Build history of the part. All positions in model axes, mm. A direction names the side the tool comes from. Give positions to 0.01 mm unless a question says otherwise; leave off trailing zeros. Order: outer loops, then holes, each group sorted by start corner. A loop starts at its lowest first (then second) coordinate and runs counter-clockwise, first axis right, second up. Notation, with made-up numbers: (68, 29.25) - (123, 29.25) arc R33 ccw to (123, 61.25) - close; hole circle Ø11 at (48.25, 28). An arc over 180 degrees is marked (long way). Write each question's results on one line, items separated by ' | '. Start each with the question number.
1) Cut at B-B on y = 35. List the corners of the cut face in (x, z).
2) Two-plate mould, pull along Y, no slides. Class faces 1 (the face through (54, 0, -16)), 2 (the face through (53, 39.37, 2)), 3 (the face through (50.78, 23.7, 1.88)): +Y half, -Y half, draft (parallel to the pull), parting line (faces both ways), or undercut.
3) Drill centre lines: line 1 along Y through (x, z) = (53.34, 2.1); line 2 along Z through (x, y) = (18, 6). Where is each one in solid material? Low to high. Write a range as from..to.
4) Drop flat-ended pins along their axis: pin 1 Ø8 at (x, y) = (25.5, 24) entering from -Z; pin 2 Ø1 at (x, z) = (41, -31) entering from +Y. Give the stop position or say it passes through.
5) Cut at C-C on x = 7.5. List the corners of the cut face in (y, z).
6) Cut at A-A on x = 53.34. List the corners of the cut face in (y, z).
7) Tool access for faces 4 (the face through (0, 10.8, 0.3)), 5 (the face through (53, 25, 0)): list every direction of +Z, -Z, +X, -X, +Y, -Y with a clear straight run to the whole face (end or side of a thin tool).
Autodesk Inventor part; units mm, degrees
ref_plane "YZ Plane" through (0, 0, 0) normal (1, 0, 0) x (0, 1, 0)
ref_plane "XZ Plane" through (0, 0, 0) normal (0, 1, 0) x (-1, 0, 0)
ref_plane "XY Plane" through (0, 0, 0) normal (0, 0, 1) x (1, 0, 0)
sketch "Sketch1" plane through (0, 0, 0) normal (0, 1, 0) x (-1, 0, 0)
  line L0 (0, 0) -> (0, -35.56)
  line L1 (0, -35.56) -> (-106.68, -35.56)
  line L2 (-106.68, -35.56) -> (-106.68, 0)
  line L3 (0, 0) -> (0, 3.81)
  line L4 (0, 3.81) -> (-106.68, 3.81)
  line L5 (-106.68, 3.81) -> (-106.68, 0)
  dimension "d0" = 35.56
  dimension "d1" = 106.68
  dimension "d2" = 3.81
extrude "Extrusion1" add sketch "Sketch1" along normal blind 3.81
sketch "Sketch2" plane through (0, 3.81, 0) normal (0, 1, 0) x (1, 0, 0)
  line L0 (0, 35.56) -> (0, -3.81)
  line L1 (0, -3.81) -> (0, 0)
  line L2 (0, 0) -> (106.68, 0)
  line L3 (106.68, -3.81) -> (106.68, 35.56)
  line L4 (106.68, -3.81) -> (0, -3.81)
extrude "Extrusion2" add sketch "Sketch2" along normal blind 35.56
sketch "Sketch3" plane through (106.68, 3.81, 0) normal (0, 0, -1) x (-1, 0, 0)
  line L0 (106.68, -3.81) -> (106.68, 35.56)
  line L1 (106.68, 15.875) -> (0, 15.875)
  line L2 (0, -3.81) -> (0, 35.56)
  circle A0 centre (53.34, 15.875) radius 4.7625
  dimension "d10" = 9.525
extrude "Extrusion3" cut sketch "Sketch3" against normal blind 17.4625
properties part number "Flywheel top lift wheel bracket" material "Steel, Alloy"
Results:
1) outline: (0, 0) - (106.68, 0) - (106.68, 3.81) - (0, 3.81) - close
2) face 1: -Y half | face 2: +Y half | face 3: undercut
3) line 1: 0..14.92, 24.45..39.37 | line 2: 0..3.81
4) pin 1: z = 0 | pin 2: y = 3.81
5) outline: (0, -35.56) - (3.81, -35.56) - (3.81, 0) - (39.37, 0) - (39.37, 3.81) - (0, 3.81) - close
6) outline: (0, -35.56) - (3.81, -35.56) - (3.81, 0) - (14.92, 0) - (14.92, 3.81) - (0, 3.81) - close; (24.45, 0) - (39.37, 0) - (39.37, 3.81) - (24.45, 3.81) - close
7) face 4: +Z, -Z, -X, +Y, -Y | face 5: -Z, +X, -X, +Y
